from build123d import *

# Parameters (mm, degrees)
F0_W     = 150
F0_H     = 76
F0_W_2   = 35
F0_H_2   = 35
F1_DEPTH = 2
F2_DEPTH = 4
F3_R     = 1.99999


# Not quite as in the source:
# - a fillet or chamfer is up to 0.001 mm smaller than in the source, because OpenCascade refuses the exact size


with BuildPart() as f1:
    # F0 (on Front) → F1 (new body)
    with BuildSketch(Plane.XZ):
        Rectangle(F0_W, F0_H)
        with Locations((-55.5, -18.5)):
            Rectangle(F0_W_2, F0_H_2, mode=Mode.SUBTRACT)
        with Locations((-18.5, -18.5)):
            Rectangle(F0_W_2, F0_H_2, mode=Mode.SUBTRACT)
        with Locations((18.5, -18.5)):
            Rectangle(F0_W_2, F0_H_2, mode=Mode.SUBTRACT)
        with Locations((55.5, -18.5)):
            Rectangle(F0_W_2, F0_H_2, mode=Mode.SUBTRACT)
        with Locations((-55.5, 18.5)):
            Rectangle(F0_W_2, F0_H_2, mode=Mode.SUBTRACT)
        with Locations((-18.5, 18.5)):
            Rectangle(F0_W_2, F0_H_2, mode=Mode.SUBTRACT)
        with Locations((18.5, 18.5)):
            Rectangle(F0_W_2, F0_H_2, mode=Mode.SUBTRACT)
        with Locations((55.5, 18.5)):
            Rectangle(F0_W_2, F0_H_2, mode=Mode.SUBTRACT)
        with Locations((-55.5, -18.5)):
            Rectangle(F0_W_2, F0_H_2)
        with Locations((-55.5, 18.5)):
            Rectangle(F0_W_2, F0_H_2)
        with Locations((-18.5, 18.5)):
            Rectangle(F0_W_2, F0_H_2)
        with Locations((18.5, 18.5)):
            Rectangle(F0_W_2, F0_H_2)
        with Locations((55.5, -18.5)):
            Rectangle(F0_W_2, F0_H_2)
        with Locations((55.5, 18.5)):
            Rectangle(F0_W_2, F0_H_2)
        with Locations((18.5, -18.5)):
            Rectangle(F0_W_2, F0_H_2)
        with Locations((-18.5, -18.5)):
            Rectangle(F0_W_2, F0_H_2)
    extrude(amount=F1_DEPTH)

    # F0 (on Front) → F2 (join)
    with BuildSketch(Plane.XZ):
        Rectangle(F0_W, F0_H)
        with Locations((-55.5, -18.5)):
            Rectangle(F0_W_2, F0_H_2, mode=Mode.SUBTRACT)
        with Locations((-18.5, -18.5)):
            Rectangle(F0_W_2, F0_H_2, mode=Mode.SUBTRACT)
        with Locations((18.5, -18.5)):
            Rectangle(F0_W_2, F0_H_2, mode=Mode.SUBTRACT)
        with Locations((55.5, -18.5)):
            Rectangle(F0_W_2, F0_H_2, mode=Mode.SUBTRACT)
        with Locations((-55.5, 18.5)):
            Rectangle(F0_W_2, F0_H_2, mode=Mode.SUBTRACT)
        with Locations((-18.5, 18.5)):
            Rectangle(F0_W_2, F0_H_2, mode=Mode.SUBTRACT)
        with Locations((18.5, 18.5)):
            Rectangle(F0_W_2, F0_H_2, mode=Mode.SUBTRACT)
        with Locations((55.5, 18.5)):
            Rectangle(F0_W_2, F0_H_2, mode=Mode.SUBTRACT)
    extrude(amount=F2_DEPTH)

    # F3 (radius 2 in the source; OpenCascade refuses exactly that, so slightly less here)
    f3_edges = [f1.edges().sort_by_distance(p)[0] for p in [
        (-73, -2, -18.5),
        (-55.5, -2, -1),
        (-55.5, -2, 36),
        (-36, -2, 18.5),
        (-18.5, -2, 36),
        (-73, -2, 18.5),
        (1, -2, 18.5),
        (18.5, -2, 36),
        (38, -2, 18.5),
        (55.5, -2, 36),
        (55.5, -2, -1),
        (38, -2, -18.5),
        (18.5, -2, -1),
        (1, -2, -18.5),
        (-18.5, -2, -1),
        (-36, -2, -18.5),
        (73, -2, -18.5),
        (55.5, -2, -36),
        (18.5, -2, -36),
        (-18.5, -2, -36),
        (-55.5, -2, -36),
        (-38, -2, -18.5),
        (-1, -2, -18.5),
        (36, -2, -18.5),
        (55.5, -2, 1),
        (73, -2, 18.5),
        (18.5, -2, 1),
        (36, -2, 18.5),
        (-18.5, -2, 1),
        (-1, -2, 18.5),
        (-55.5, -2, 1),
        (-38, -2, 18.5),
    ]]
    fillet(f3_edges, radius=F3_R)


solid = f1.part
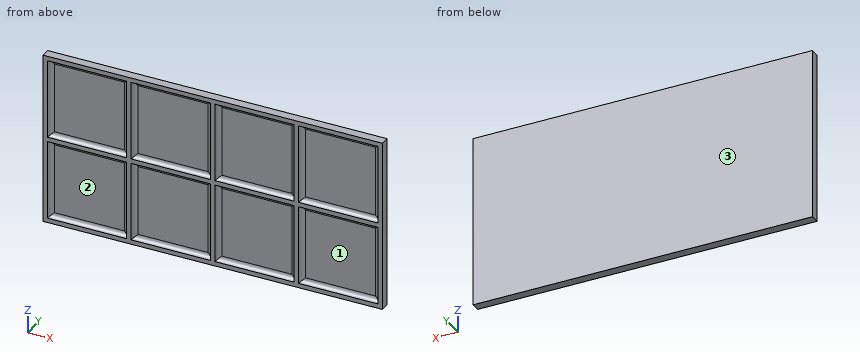
The model under review builds one solid part; all positions refer to its coordinate system, in mm. Face numbers are marked on the shaded views. Give positions to 0.01 mm unless a question says otherwise; leave off trailing zeros.
1. Draft analysis for pull direction X (two halves, no side actions). For the marked faces 1, 2 and 3, state which applies: +X half, -X half, draft (parallel to the pull), parting line (faces both ways), or undercut.
2. For P1, Ø9.5, axis at x = 51.5, z = -19, coming from the -Y side, flat-tipped, find the tip position at first contact; note if it passes through.
3. Add section C-C, the plane y = -2.95. Count the separate pieces of the cut face and the enclosed holes in it, plus the area to 3 significant figures.
4. Wall thickness on L1, parallel to X at y = -3.7, z = -2.5; L2, parallel to X at y = -2.65, z = 15; L3, parallel to Z at x = -5, y = -3.55: over which ranges is each line inside the solid? List them lowest first.
Worked answers:
1. face 1: undercut
1. face 2: undercut
1. face 3: draft
2. P1: stops at y = -2
3. separate pieces: 1
3. enclosed holes: 8
3. area: 1,930 mm2
4. L1: x = -75 to -72.98, -38.02 to -35.98, -1.02 to 1.02, 35.98 to 38.02, 72.98 to 75
4. L2: x = -75 to -72.48, -38.52 to -35.48, -1.52 to 1.52, 35.48 to 38.52, 72.48 to 75
4. L3: z = -38 to -35.95, -1.05 to 1.05, 35.95 to 38
